Build history of the part. All positions in model axes, mm. A direction names the side the tool comes from. Coordinates: 2 decimals unless noted, no trailing zeros. Loops run counter-clockwise (first coordinate to the right, second up) from the corner with the lowest first, then second, coordinate; pieces in that order, holes last.
Item 1: Cut at C-C (x = -24). List the corners of the cut face in (y, z), and give its area (3 significant figures).
Item 2: Cut at A-A (y = 25). List the corners of the cut face in (x, z), and give its area (3 significant figures).
Item 3: Flat gauge pin, fed straight in: pin 1 (10 mm diameter, centred on x = -5, z = -3, fed in from +Y). Where does the tip first touch, or does it go through?
Item 4: Cut at B-B (z = 22). List the corners of the cut face in (x, y).
Item 5: 3-axis set-ups, long thin cutter, end or side, ignore diameter. For faces 4 (the face through (-1, 36, 69.117)), 5 (the face through (-1, 6.35, 21)), 6 (the face through (42.626, 90.247, 25.29)): which of +Z, -Z, +X, -X, +Y, -Y reach the whole face in a straight line?
Item 6: Drill centre lines: line 1 along X through (y, z) = (25, 4); line 2 along Z through (x, y) = (19.5, 55); line 3 along Y through (x, z) = (-40, 13.5). Where is each one in solid material? Low to high.
Item 7: Mould opens along X. For faces 1 (the face through (47.366, 47, 22)), 2 (the face through (-43.1, 90.38, 25.29)), 3 (the face through (-1, 0, 21)) say: released by +X, released by -X, zero draft, split by the parting line, or undercut.
from build123d import *

# Parameters (mm, degrees)
SKETCH1_W           = 95.25
SKETCH1_H           = 95.25
BOSS_EXTRUDE1_DEPTH = 95.25
SHELL1_T            = -6.35
CUT_EXTRUDE1_DEPTH  = 88.9


with BuildPart() as part:
    # Sketch1 → Boss-Extrude1 (new body)
    with BuildSketch(Plane(origin=(0, 0, 0), x_dir=(1, 0, 0), z_dir=(0, 1, 0))):
        with Locations((-0.25880421, -21.492307692)):
            Rectangle(SKETCH1_W, SKETCH1_H)
    extrude(amount=BOSS_EXTRUDE1_DEPTH)

    # Shell1
    shell1_openings = [part.faces().sort_by_distance(p)[0] for p in [
        (-0.25880421, 95.25, 21.492307692),
    ]]
    offset(amount=SHELL1_T, openings=shell1_openings, kind=Kind.INTERSECTION)

    # Sketch2 → Cut-Extrude1 (cut)
    with BuildSketch(Plane.XY.offset(69.117307692)):
        Polygon((41.01619579, 95.25), (-41.53380421, 95.25), (-44.70880421, 85.381498792), (44.19119579, 85.381498792), align=None)
    extrude(amount=-CUT_EXTRUDE1_DEPTH, mode=Mode.SUBTRACT)


solid = part.part
Filled sheet:
1. outline: (0, -26.13) - (95.25, -26.13) - (95.25, -19.78) - (6.35, -19.78) - (6.35, 62.77) - (85.38, 62.77) - (85.38, 69.12) - (0, 69.12) - close
1. area: 1,670 mm2
2. outline: (-47.88, -26.13) - (47.37, -26.13) - (47.37, 69.12) - (-47.88, 69.12) - close; hole (-41.53, -19.78) - (41.02, -19.78) - (41.02, 62.77) - (-41.53, 62.77) - close
2. area: 2,260 mm2
3. pin 1: stops at y = 6.35
4. outline: (-47.88, 0) - (47.37, 0) - (47.37, 95.25) - (41.02, 95.25) - (44.19, 85.38) - (41.02, 85.38) - (41.02, 6.35) - (-41.53, 6.35) - (-41.53, 85.38) - (-44.71, 85.38) - (-41.53, 95.25) - (-47.88, 95.25) - close
5. face 4: +Z, +X, -X, +Y, -Y
5. face 5: +Y
5. face 6: +Z
6. line 1: x = -47.88 to -41.53, 41.02 to 47.37
6. line 2: z = -26.13 to -19.78, 62.77 to 69.12
6. line 3: y = 0 to 6.35
7. face 1: released by +X
7. face 2: undercut
7. face 3: zero draft
